Check sheet for the modelled part. Datum: model origin and axes. Units: mm. Give positions to 0.01 mm unless a question says otherwise; leave off trailing zeros. Write each loop counter-clockwise with the first axis right and the second up, starting at its lowest first coordinate (ties: lowest second). Pieces come first, ordered by that corner, then holes. Notation, with made-up numbers: M -38,22 L -10,22 A25 cw -10,60 Z; hole C 48,2.5 d10. An arc over 180 degrees is marked long. Write item = value, one per line. Start each with the question number.
1) Cross-section at A-A, the plane z = 55. Record the cut outline in (x, y), plus the area to 3 significant figures.
2) Scan lines: line 1 along Z through (x, y) = (2, 33.5); line 2 along Z through (x, y) = (2, 26.5); line 3 along X through (y, z) = (28, 135). Record each from-to range of solid material in increasing order. Write a range as [from, to].
3) Go/stop test with flat-tipped pins: pin 1 (5 mm diameter, centred on x = 0, z = 15, fed in from -Y); pin 2 (7.5 mm diameter, centred on x = 0, z = 135, fed in from +Y); pin 3 (11 mm diameter, centred on x = 0, z = 15, fed in from +Y); pin 4 (4 mm diameter, centred on x = 1.5, z = 54.5, fed in from +Y). Record where each tip stops, or that it passes through.
4) Cross-section at B-B, the plane x = 0. Give the number of separate pieces and of enclosed holes in the cut face, plus the area to 3 significant figures.
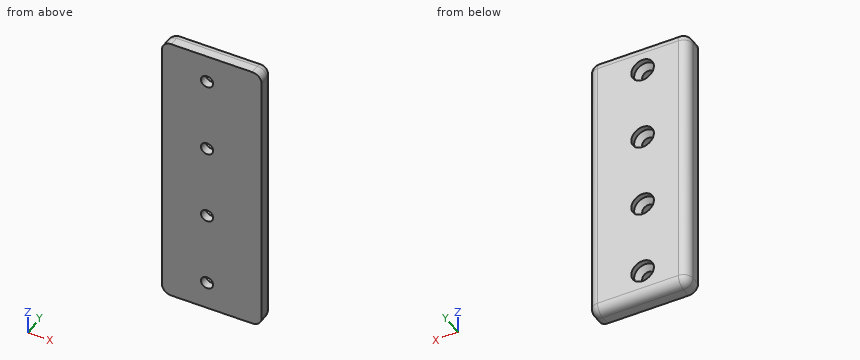
```python
from build123d import *

# Parameters (mm, degrees)
SKETCH1_W               = 48
SKETCH1_H               = 48
SKETCH1_R               = 13.75
SKETCH1_H_2             = 10
BOSS_EXTRUDE1_DEPTH     = 230
SKETCH3_R               = 6
CUT_EXTRUDE1_DEPTH      = 0.5
SKETCH4_R               = 3.25
CUT_EXTRUDE2_DEPTH      = 240.26061105
CUT_EXTRUDE3_REACH      = 241.261
CUT_EXTRUDE3_END_RADIUS = 13.75
SKETCH5_R               = 6.5
CUT_EXTRUDE4_REACH      = 243.738
CUT_EXTRUDE4_END_RADIUS = 13.75
CUT_EXTRUDE4_START      = -5
CHAMFER1_SIZE           = 5
SKETCH8_W               = 230
SKETCH8_H               = 1.2
CUT_EXTRUDE5_DEPTH      = 10
SKETCH9_W               = 53
SKETCH9_H               = 80
CUT_EXTRUDE6_DEPTH      = 233.036635039
FILLET2_R               = 5


with BuildPart() as part:
    # Sketch1 → Boss-Extrude1 (new body)
    # profile 1 of 3: a face of its own
    with BuildSketch(Plane.XY):
        Rectangle(SKETCH1_W, SKETCH1_H)
        Circle(SKETCH1_R, mode=Mode.SUBTRACT)
    # profile 2 of 3: a face of its own
    with BuildSketch(Plane.XY):
        with Locations((0, 30.2)):
            Rectangle(SKETCH1_W, SKETCH1_H_2)
    # profile 3 of 3: a face of its own
    with BuildSketch(Plane.XY):
        Polygon((24, 24), (24, -24), (29, -24), (29, 35.2), (24, 35.2), (24, 25.2), align=None)
    extrude(amount=BOSS_EXTRUDE1_DEPTH)

    # Sketch3 → Cut-Extrude1 (cut)
    with BuildSketch(Plane(origin=(0, 35.2, 0), x_dir=(1, 0, 0), z_dir=(0, 1, 0))):
        with Locations(Location((0, -15, 0), (0, 0, 270))):
            Circle(SKETCH3_R)
        with Locations(Location((0, -55, 0), (0, 0, 270))):
            Circle(SKETCH3_R)
        with Locations(Location((0, -95, 0), (0, 0, 270))):
            Circle(SKETCH3_R)
        with Locations(Location((0, -135, 0), (0, 0, 270))):
            Circle(SKETCH3_R)
        with Locations(Location((0, -175, 0), (0, 0, 270))):
            Circle(SKETCH3_R)
        with Locations(Location((0, -215, 0), (0, 0, 270))):
            Circle(SKETCH3_R)
    extrude(amount=-CUT_EXTRUDE1_DEPTH, mode=Mode.SUBTRACT)

    # Sketch4 → Cut-Extrude2 (cut, through all)
    with BuildSketch(Plane(origin=(0, 35.2, 0), x_dir=(1, 0, 0), z_dir=(0, 1, 0))):
        with Locations(Location((0, -15, 0), (0, 0, 270))):
            Circle(SKETCH4_R)
        with Locations(Location((0, -55, 0), (0, 0, 270))):
            Circle(SKETCH4_R)
        with Locations(Location((0, -95, 0), (0, 0, 270))):
            Circle(SKETCH4_R)
        with Locations(Location((0, -135, 0), (0, 0, 270))):
            Circle(SKETCH4_R)
        with Locations(Location((0, -175, 0), (0, 0, 270))):
            Circle(SKETCH4_R)
        with Locations(Location((0, -215, 0), (0, 0, 270))):
            Circle(SKETCH4_R)
    extrude(amount=-CUT_EXTRUDE2_DEPTH, mode=Mode.SUBTRACT)

    # Cut-Extrude3: up to this cylinder (the profile starts outside it)
    cut_extrude3_end = Plane(origin=(0, 0, 115), z_dir=(0, 0, -1)) * Cylinder(CUT_EXTRUDE3_END_RADIUS, 711.022, mode=Mode.PRIVATE)
    # Sketch5 → Cut-Extrude3 (cut, up to the surface)
    with BuildSketch(Plane.XZ.offset(24), mode=Mode.PRIVATE) as cut_extrude3_sk1:
        with Locations(Location((0, 215, 0), (0, 0, 270))):
            Circle(SKETCH5_R)
    cut_extrude3_tool1 = extrude(cut_extrude3_sk1.sketch, amount=-CUT_EXTRUDE3_REACH, mode=Mode.PRIVATE) - cut_extrude3_end
    add(cut_extrude3_tool1.solids().sort_by_distance((0, -24, 215))[0], mode=Mode.SUBTRACT)
    # Sketch5 → Cut-Extrude3 (cut, up to the surface)
    with BuildSketch(Plane.XZ.offset(24), mode=Mode.PRIVATE) as cut_extrude3_sk2:
        with Locations(Location((0, 175, 0), (0, 0, 270))):
            Circle(SKETCH5_R)
    cut_extrude3_tool2 = extrude(cut_extrude3_sk2.sketch, amount=-CUT_EXTRUDE3_REACH, mode=Mode.PRIVATE) - cut_extrude3_end
    add(cut_extrude3_tool2.solids().sort_by_distance((0, -24, 175))[0], mode=Mode.SUBTRACT)
    # Sketch5 → Cut-Extrude3 (cut, up to the surface)
    with BuildSketch(Plane.XZ.offset(24), mode=Mode.PRIVATE) as cut_extrude3_sk3:
        with Locations(Location((0, 135, 0), (0, 0, 270))):
            Circle(SKETCH5_R)
    cut_extrude3_tool3 = extrude(cut_extrude3_sk3.sketch, amount=-CUT_EXTRUDE3_REACH, mode=Mode.PRIVATE) - cut_extrude3_end
    add(cut_extrude3_tool3.solids().sort_by_distance((0, -24, 135))[0], mode=Mode.SUBTRACT)
    # Sketch5 → Cut-Extrude3 (cut, up to the surface)
    with BuildSketch(Plane.XZ.offset(24), mode=Mode.PRIVATE) as cut_extrude3_sk4:
        with Locations(Location((0, 95, 0), (0, 0, 270))):
            Circle(SKETCH5_R)
    cut_extrude3_tool4 = extrude(cut_extrude3_sk4.sketch, amount=-CUT_EXTRUDE3_REACH, mode=Mode.PRIVATE) - cut_extrude3_end
    add(cut_extrude3_tool4.solids().sort_by_distance((0, -24, 95))[0], mode=Mode.SUBTRACT)
    # Sketch5 → Cut-Extrude3 (cut, up to the surface)
    with BuildSketch(Plane.XZ.offset(24), mode=Mode.PRIVATE) as cut_extrude3_sk5:
        with Locations(Location((0, 55, 0), (0, 0, 270))):
            Circle(SKETCH5_R)
    cut_extrude3_tool5 = extrude(cut_extrude3_sk5.sketch, amount=-CUT_EXTRUDE3_REACH, mode=Mode.PRIVATE) - cut_extrude3_end
    add(cut_extrude3_tool5.solids().sort_by_distance((0, -24, 55))[0], mode=Mode.SUBTRACT)
    # Sketch5 → Cut-Extrude3 (cut, up to the surface)
    with BuildSketch(Plane.XZ.offset(24), mode=Mode.PRIVATE) as cut_extrude3_sk6:
        with Locations(Location((0, 15, 0), (0, 0, 270))):
            Circle(SKETCH5_R)
    cut_extrude3_tool6 = extrude(cut_extrude3_sk6.sketch, amount=-CUT_EXTRUDE3_REACH, mode=Mode.PRIVATE) - cut_extrude3_end
    add(cut_extrude3_tool6.solids().sort_by_distance((0, -24, 15))[0], mode=Mode.SUBTRACT)

    # Cut-Extrude4: up to this cylinder (the profile starts outside it)
    cut_extrude4_end = Plane(origin=(0, 0, 115), z_dir=(0, 0, -1)) * Cylinder(CUT_EXTRUDE4_END_RADIUS, 715.976, mode=Mode.PRIVATE)
    # Sketch7 → Cut-Extrude4 (cut, up to the surface)
    with BuildSketch(Plane(origin=(0, 24, 0), x_dir=(1, 0, 0), z_dir=(0, 1, 0)).offset(CUT_EXTRUDE4_START), mode=Mode.PRIVATE) as cut_extrude4_sk1:
        Polygon((0, -8.533676985), (-5.6, -11.766838493), (-5.6, -18.233161507), (0, -21.466323015), (5.6, -18.233161507), (5.6, -11.766838493), align=None)
    cut_extrude4_tool1 = extrude(cut_extrude4_sk1.sketch, amount=-CUT_EXTRUDE4_REACH, mode=Mode.PRIVATE) - cut_extrude4_end
    add(cut_extrude4_tool1.solids().sort_by_distance((0, 19, 15))[0], mode=Mode.SUBTRACT)
    # Sketch7 → Cut-Extrude4 (cut, up to the surface)
    with BuildSketch(Plane(origin=(0, 24, 0), x_dir=(1, 0, 0), z_dir=(0, 1, 0)).offset(CUT_EXTRUDE4_START), mode=Mode.PRIVATE) as cut_extrude4_sk2:
        Polygon((0, -48.533676985), (-5.6, -51.766838493), (-5.6, -58.233161507), (0, -61.466323015), (5.6, -58.233161507), (5.6, -51.766838493), align=None)
    cut_extrude4_tool2 = extrude(cut_extrude4_sk2.sketch, amount=-CUT_EXTRUDE4_REACH, mode=Mode.PRIVATE) - cut_extrude4_end
    add(cut_extrude4_tool2.solids().sort_by_distance((0, 19, 55))[0], mode=Mode.SUBTRACT)
    # Sketch7 → Cut-Extrude4 (cut, up to the surface)
    with BuildSketch(Plane(origin=(0, 24, 0), x_dir=(1, 0, 0), z_dir=(0, 1, 0)).offset(CUT_EXTRUDE4_START), mode=Mode.PRIVATE) as cut_extrude4_sk3:
        Polygon((0, -88.533676985), (-5.6, -91.766838493), (-5.6, -98.233161507), (0, -101.466323015), (5.6, -98.233161507), (5.6, -91.766838493), align=None)
    cut_extrude4_tool3 = extrude(cut_extrude4_sk3.sketch, amount=-CUT_EXTRUDE4_REACH, mode=Mode.PRIVATE) - cut_extrude4_end
    add(cut_extrude4_tool3.solids().sort_by_distance((0, 19, 95))[0], mode=Mode.SUBTRACT)
    # Sketch7 → Cut-Extrude4 (cut, up to the surface)
    with BuildSketch(Plane(origin=(0, 24, 0), x_dir=(1, 0, 0), z_dir=(0, 1, 0)).offset(CUT_EXTRUDE4_START), mode=Mode.PRIVATE) as cut_extrude4_sk4:
        Polygon((0, -128.533676985), (-5.6, -131.766838493), (-5.6, -138.233161507), (0, -141.466323015), (5.6, -138.233161507), (5.6, -131.766838493), align=None)
    cut_extrude4_tool4 = extrude(cut_extrude4_sk4.sketch, amount=-CUT_EXTRUDE4_REACH, mode=Mode.PRIVATE) - cut_extrude4_end
    add(cut_extrude4_tool4.solids().sort_by_distance((0, 19, 135))[0], mode=Mode.SUBTRACT)
    # Sketch7 → Cut-Extrude4 (cut, up to the surface)
    with BuildSketch(Plane(origin=(0, 24, 0), x_dir=(1, 0, 0), z_dir=(0, 1, 0)).offset(CUT_EXTRUDE4_START), mode=Mode.PRIVATE) as cut_extrude4_sk5:
        Polygon((0, -168.533676985), (-5.6, -171.766838493), (-5.6, -178.233161507), (0, -181.466323015), (5.6, -178.233161507), (5.6, -171.766838493), align=None)
    cut_extrude4_tool5 = extrude(cut_extrude4_sk5.sketch, amount=-CUT_EXTRUDE4_REACH, mode=Mode.PRIVATE) - cut_extrude4_end
    add(cut_extrude4_tool5.solids().sort_by_distance((0, 19, 175))[0], mode=Mode.SUBTRACT)
    # Sketch7 → Cut-Extrude4 (cut, up to the surface)
    with BuildSketch(Plane(origin=(0, 24, 0), x_dir=(1, 0, 0), z_dir=(0, 1, 0)).offset(CUT_EXTRUDE4_START), mode=Mode.PRIVATE) as cut_extrude4_sk6:
        Polygon((0, -208.533676985), (-5.6, -211.766838493), (-5.6, -218.233161507), (0, -221.466323015), (5.6, -218.233161507), (5.6, -211.766838493), align=None)
    cut_extrude4_tool6 = extrude(cut_extrude4_sk6.sketch, amount=-CUT_EXTRUDE4_REACH, mode=Mode.PRIVATE) - cut_extrude4_end
    add(cut_extrude4_tool6.solids().sort_by_distance((0, 19, 215))[0], mode=Mode.SUBTRACT)

    # Chamfer1
    # the kernel refuses this chamfer: 5 mm, written as the material it takes off along each edge
    with BuildSketch(Plane(origin=(0, 34.7, 215), x_dir=(0, 0, 1), z_dir=(-1, 0, 0))) as chamfer1_piece_1_section:
        Polygon((3.25, -CHAMFER1_SIZE), (3.25 + CHAMFER1_SIZE, 0), (3.25, 0), align=None)
    chamfer1_piece_1 = revolve(axis=Axis((0, 34.7, 215), (0, 1, 0)), mode=Mode.PRIVATE)
    chamfer1_piece_1 = chamfer1_piece_1 & Plane(origin=(0, 31.051548399, 215), x_dir=(0, 0, 1), z_dir=(0, 1, 0)) * Cylinder(6, 33, mode=Mode.PRIVATE)
    add(chamfer1_piece_1, mode=Mode.SUBTRACT)
    with BuildSketch(Plane(origin=(0, 34.7, 175), x_dir=(0, 0, 1), z_dir=(-1, 0, 0))) as chamfer1_piece_2_section:
        Polygon((3.25, -CHAMFER1_SIZE), (3.25 + CHAMFER1_SIZE, 0), (3.25, 0), align=None)
    chamfer1_piece_2 = revolve(axis=Axis((0, 34.7, 175), (0, 1, 0)), mode=Mode.PRIVATE)
    chamfer1_piece_2 = chamfer1_piece_2 & Plane(origin=(0, 31.051548399, 175), x_dir=(0, 0, 1), z_dir=(0, 1, 0)) * Cylinder(6, 33, mode=Mode.PRIVATE)
    add(chamfer1_piece_2, mode=Mode.SUBTRACT)
    with BuildSketch(Plane(origin=(0, 34.7, 135), x_dir=(0, 0, 1), z_dir=(-1, 0, 0))) as chamfer1_piece_3_section:
        Polygon((3.25, -CHAMFER1_SIZE), (3.25 + CHAMFER1_SIZE, 0), (3.25, 0), align=None)
    chamfer1_piece_3 = revolve(axis=Axis((0, 34.7, 135), (0, 1, 0)), mode=Mode.PRIVATE)
    chamfer1_piece_3 = chamfer1_piece_3 & Plane(origin=(0, 31.051548399, 135), x_dir=(0, 0, 1), z_dir=(0, 1, 0)) * Cylinder(6, 33, mode=Mode.PRIVATE)
    add(chamfer1_piece_3, mode=Mode.SUBTRACT)
    with BuildSketch(Plane(origin=(0, 34.7, 95), x_dir=(0, 0, 1), z_dir=(-1, 0, 0))) as chamfer1_piece_4_section:
        Polygon((3.25, -CHAMFER1_SIZE), (3.25 + CHAMFER1_SIZE, 0), (3.25, 0), align=None)
    chamfer1_piece_4 = revolve(axis=Axis((0, 34.7, 95), (0, 1, 0)), mode=Mode.PRIVATE)
    chamfer1_piece_4 = chamfer1_piece_4 & Plane(origin=(0, 31.051548399, 95), x_dir=(0, 0, 1), z_dir=(0, 1, 0)) * Cylinder(6, 33, mode=Mode.PRIVATE)
    add(chamfer1_piece_4, mode=Mode.SUBTRACT)
    with BuildSketch(Plane(origin=(0, 34.7, 55), x_dir=(0, 0, 1), z_dir=(-1, 0, 0))) as chamfer1_piece_5_section:
        Polygon((3.25, -CHAMFER1_SIZE), (3.25 + CHAMFER1_SIZE, 0), (3.25, 0), align=None)
    chamfer1_piece_5 = revolve(axis=Axis((0, 34.7, 55), (0, 1, 0)), mode=Mode.PRIVATE)
    chamfer1_piece_5 = chamfer1_piece_5 & Plane(origin=(0, 31.051548399, 55), x_dir=(0, 0, 1), z_dir=(0, 1, 0)) * Cylinder(6, 33, mode=Mode.PRIVATE)
    add(chamfer1_piece_5, mode=Mode.SUBTRACT)
    with BuildSketch(Plane(origin=(0, 34.7, 15), x_dir=(0, 0, 1), z_dir=(-1, 0, 0))) as chamfer1_piece_6_section:
        Polygon((3.25, -CHAMFER1_SIZE), (3.25 + CHAMFER1_SIZE, 0), (3.25, 0), align=None)
    chamfer1_piece_6 = revolve(axis=Axis((0, 34.7, 15), (0, 1, 0)), mode=Mode.PRIVATE)
    chamfer1_piece_6 = chamfer1_piece_6 & Plane(origin=(0, 31.051548399, 15), x_dir=(0, 0, 1), z_dir=(0, 1, 0)) * Cylinder(6, 33, mode=Mode.PRIVATE)
    add(chamfer1_piece_6, mode=Mode.SUBTRACT)

    # Sketch8 → Cut-Extrude5 (cut)
    with BuildSketch(Plane.ZY.offset(-24)):
        with Locations((115, 24.6)):
            Rectangle(SKETCH8_W, SKETCH8_H)
    extrude(amount=-CUT_EXTRUDE5_DEPTH, mode=Mode.SUBTRACT)


with BuildPart() as body_2:
    # of the pieces the cut leaves, the one that is kept (cut_extrude5_keep)
    add(part.part.solids().sort_by_distance((29, 25.2, 0))[0])

    # Sketch9 → Cut-Extrude6 (cut, through all)
    with BuildSketch(Plane(origin=(0, 35.2, 0), x_dir=(1, 0, 0), z_dir=(0, 1, 0))):
        with Locations((2.5, -190)):
            Rectangle(SKETCH9_W, SKETCH9_H)
    extrude(amount=-CUT_EXTRUDE6_DEPTH, mode=Mode.SUBTRACT)

    # Fillet2
    fillet2_edges = [body_2.edges().sort_by_distance(p)[0] for p in [
        (29, 30.2, 0),
        (-24, 30.2, 0),
        (2.5, 35.2, 0),
        (-24, 35.2, 75),
        (29, 35.2, 75),
        (2.5, 35.2, 150),
        (-24, 30.2, 150),
        (29, 30.2, 150),
    ]]
    fillet(fillet2_edges, radius=FILLET2_R)


solid = body_2.part
```
Reply:
q1.outline = M -24,25.2 L -3.25,25.2 L -3.25,29.7 L -6,32.45 L -6,35.2 L -19,35.2 A5 ccw -24,30.2 Z; M 3.25,25.2 L 29,25.2 L 29,30.2 A5 ccw 24,35.2 L 6,35.2 L 6,32.45 L 3.25,29.7 Z
q1.area = 432 mm2
q2.line_1 = [1.24, 9.34], [20.66, 49.34], [60.66, 89.34], [100.66, 129.34], [140.66, 148.76]
q2.line_2 = [0, 12.44], [17.56, 52.44], [57.56, 92.44], [97.56, 132.44], [137.56, 150]
q2.line_3 = [-24, -3.25], [3.25, 29]
q3.pin_1 = through
q3.pin_2 = 30.2
q3.pin_3 = 31.95
q3.pin_4 = 30.03
q4.separate_pieces = 5
q4.enclosed_holes = 0
q4.area = 1,140 mm2
